Autodesk Inventor part; units mm, degrees
ref_plane "YZ Plane" through (0, 0, 0) normal (1, 0, 0) x (0, 1, 0)
ref_plane "XZ Plane" through (0, 0, 0) normal (0, 1, 0) x (-1, 0, 0)
ref_plane "XY Plane" through (0, 0, 0) normal (0, 0, 1) x (1, 0, 0)
sketch "Sketch1" plane through (0, 0, 0) normal (0, 0, 1) x (1, 0, 0)
  line L0 (0, 0) -> (19, 0)
  line L1 (19, 0) -> (19, 9)
  line L2 (19, 9) -> (0, 9)
  line L3 (0, 9) -> (0, 0)
  point P0 (9.5, 9)
  dimension "d0" = 19
  dimension "d1" = 9
extrude "Extrusion1" add sketch "Sketch1" along normal blind 3
sketch "Sketch2" plane through (0, 0, 3) normal (0, 0, 1) x (1, 0, 0)
  line L0 (19, 9) -> (0, 9)
  circle A0 centre (9.5, 7.5) radius 1.5
  line L1 (11, 6) -> (8, 6)
  line L2 (8, 6) -> (8, 9)
  line L3 (8, 9) -> (11, 9)
  line L4 (11, 9) -> (11, 6)
  line L5 (11, 6) -> (8, 9) construction
  line L6 (8, 6) -> (11, 9) construction
  line L7 (12, 7.5) -> (7, 7.5)
  line L8 (7, 7.5) -> (7, 9)
  line L9 (7, 9) -> (12, 9)
  line L10 (12, 9) -> (12, 7.5)
  line L11 (12, 7.5) -> (7, 9) construction
  line L12 (7, 7.5) -> (12, 9) construction
  line L13 (8, 7.5) -> (11, 7.5)
  line L14 (11, 7.5) -> (11, 6)
  line L15 (11, 6) -> (8, 6)
  line L16 (8, 6) -> (8, 7.5)
  point P0 (0, 0)
  point P1 (9.5, 8.25)
  dimension "d4" = 3
  dimension "d5" = 1.5
  dimension "d73" = 0.75
  dimension "d74" = 5
extrude "Extrusion2" add sketch "Sketch2" along normal blind 20 contours A0 L7 | A0 L7
sketch "Sketch10" plane through (0, 0, 0) normal (-1, 0, 0) x (0, 0, 1)
  line L0 (0, 0) -> (3, 0)
  line L1 (3, 9) -> (3, 0)
  line L2 (3, 0) -> (2, 0)
  line L3 (2, 0) -> (2, 6)
  line L4 (2, 6) -> (3, 6)
  line L5 (3, 6) -> (3, 0)
  line L6 (3, 0) -> (2, 1)
  line L7 (3, 0) -> (4.4142, 0) construction
  line L8 (2, 1) -> (3, 2)
  line L9 (3, 0) -> (3, 9)
  line L10 (3, 2) -> (2, 3)
  line L11 (2, 3) -> (3, 4)
  line L12 (2, 5) -> (3, 4)
  line L13 (2, 5) -> (3, 6)
  dimension "d23" = 1
  dimension "d24" = 6
  dimension "d25" = 135
  dimension "d26" = 90
extrude "Extrusion8" cut sketch "Sketch10" against normal up to next contours L6 L8 L1 | L10 L11 L1 | L12 L13 L1
sketch "Sketch11" plane through (0, 0, 0) normal (0, -1, 0) x (1, 0, 0)
  line L0 (0, 3) -> (9.5, 3)
  line L1 (0, 3) -> (19, 3)
  line L2 (19, 3) -> (19, 2)
  line L3 (19, 2) -> (8.5, 2)
  line L4 (0, 2) -> (0, 3)
  line L5 (0, 3) -> (0, 2)
  line L6 (0, 3) -> (1.4142, 3) construction
  line L7 (19, 3) -> (0, 3)
  line L8 (9.5, 3) -> (8.5, 2)
  line L9 (9.5, 3) -> (10.9142, 3) construction
  line L10 (10.5, 2) -> (8.5, 2)
  line L11 (9.5, 3) -> (10.5, 2)
  line L12 (10.5, 2) -> (8.5, 2)
  line L13 (8.5, 2) -> (0, 2)
  line L14 (7.5, 3) -> (8.5, 2)
  line L15 (8.5, 2) -> (6.5, 2)
  line L16 (7.5, 3) -> (6.5, 2)
  line L17 (5.5, 3) -> (6.5, 2)
  line L18 (6.5, 2) -> (4.5, 2)
  line L19 (5.5, 3) -> (4.5, 2)
  line L20 (3.5, 3) -> (4.5, 2)
  line L21 (4.5, 2) -> (2.5, 2)
  line L22 (3.5, 3) -> (2.5, 2)
  line L23 (12.5, 2) -> (10.5, 2)
  line L24 (11.5, 3) -> (12.5, 2)
  line L25 (11.5, 3) -> (10.5, 2)
  line L26 (14.5, 2) -> (12.5, 2)
  line L27 (13.5, 3) -> (14.5, 2)
  line L28 (13.5, 3) -> (12.5, 2)
  line L29 (16.5, 2) -> (14.5, 2)
  line L30 (15.5, 3) -> (16.5, 2)
  line L31 (15.5, 3) -> (14.5, 2)
  point P0 (0, 0)
  dimension "d30" = 135
  dimension "d33" = 2
  dimension "d40" = 2
extrude "Extrusion9" cut sketch "Sketch11" against normal blind 6 contours L0 L22 L13 L4 | L0 L19 L20 | L0 L16 L17 | L0 L8 L14 | L1 L25 L11 | L1 L28 L24 | L1 L31 L27 | L1 L2 L3 L30
fillet "Fillet2" radius 1 4 edges at (19, 0, 1) (19, 9, 1.5) (0, 0, 1) (0, 9, 1.5)
sketch "Sketch13" plane through (9.5, 7.5, 23) normal (0, 0, 1) x (1, 0, 0)
  line L0 (9.5, -6.5) -> (9.5, 0.5)
  arc A0 (8.5, -7.5) -> (9.5, -6.5) centre (8.5, -6.5) ccw
  line L1 (-8.5, -7.5) -> (8.5, -7.5)
  arc A1 (-9.5, -6.5) -> (-8.5, -7.5) centre (-8.5, -6.5) ccw
  line L2 (-9.5, 0.5) -> (-9.5, -6.5)
  arc A2 (-8.5, 1.5) -> (-9.5, 0.5) centre (-8.5, 0.5) ccw
  line L3 (8.5, 1.5) -> (-8.5, 1.5)
  arc A3 (9.5, 0.5) -> (8.5, 1.5) centre (8.5, 0.5) ccw
  point P0 (-9.5, -7.5)
extrude "Extrusion12" add sketch "Sketch13" along normal blind 4
sketch "Sketch14" plane through (9.5, 7.5, 27) normal (0, 0, 1) x (1, 0, 0)
  line L0 (-8.5, -7.5) -> (8.5, -7.5)
  circle A0 centre (0, -4.5) radius 1.65
  point P0 (-9.5, -7.5)
  dimension "d67" = 3
  dimension "d68" = 3.3
extrude "Extrusion13" cut sketch "Sketch14" against normal up to next
extrude "Extrusion14" add sketch "Sketch2" along normal up to next contours L4 A0 L0 | A0 L2 L0 | L4 L1 A0 | A0 L1 L2
extrude "Extrusion15" add sketch "Sketch2" along normal up to next contours L10 L7 L4 L0 | L4 A0 L0 | A0 L2 L0 | A0 L7 | L2 L7 L8 L0 picked at (9.5, 8)
extrude "Extrusion16" cut sketch "Sketch2" along normal up to surface (20 mm away) contours L4 L1 A0 | A0 L7 | A0 L1 L2 picked at (9.1091, 7.1883)
properties part number "clamp-base9x19mm-SampleH20-screwM4(Miracca)"
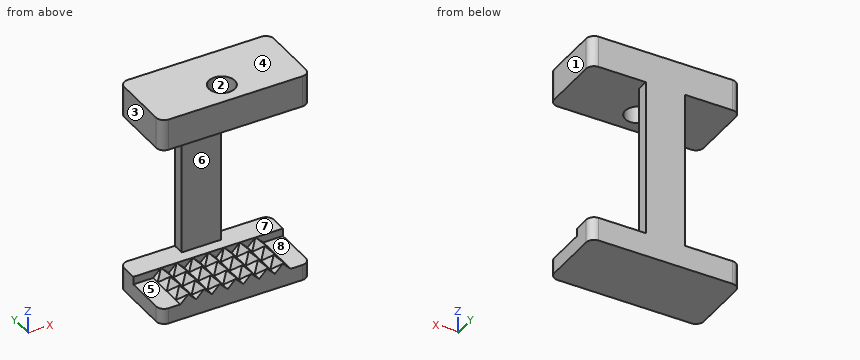
Here's how the part is built. I have some questions about the finished solid (model axes, mm). Face numbers are marked on the shaded views. A direction names the side the tool comes from. Coordinates: 2 decimals unless noted, no trailing zeros. Write each loop counter-clockwise with the first axis right and the second up, starting at its lowest first coordinate (ties: lowest second). Pieces come first, ordered by that corner, then holes. Notation, with made-up numbers: (13, 56.5) - (59, 56.5) arc R13 ccw to (59, 81.5) - close; hole circle Ø6 at (27, -11.5). An arc over 180 degrees is marked (long way). One line per item, written item: value.
1) We'd pull the mould along X, two halves only. Please class the marked faces 1, 2, 3 and 4: pulls with the +X half, pulls with the -X half, needs draft (parallel to the pull), parting line crosses it, or undercut.
Model answer:
face 1: pulls with the +X half
face 2: undercut
face 3: pulls with the -X half
face 4: needs draft
2) Suppose I cut it at A-A on z = 23.5. Write out the boundary of the cut face in (x, y), and give its area (3 significant figures).
Model answer:
outline: (0, 1) arc R1 ccw to (1, 0) - (18, 0) arc R1 ccw to (19, 1) - (19, 8) arc R1 ccw to (18, 9) - (1, 9) arc R1 ccw to (0, 8) - close; hole circle Ø3.3 at (9.5, 3)
area: 162 mm²
3) Suppose I cut it at B-B on z = 6.75. Write out the boundary of the cut face in (x, y), and give its area (3 significant figures).
Model answer:
outline: (7, 7.5) - (12, 7.5) - (12, 9) - (7, 9) - close
area: 7.50 mm²
4) I need wall thicknesses on line 1 along Z through (x, y) = (2.5, 7.5); line 2 along Z through (x, y) = (6.5, 3); line 3 along Y through (x, z) = (9.5, 25.7). Which ranges of each line are inside material? Lowest first, please.
Model answer:
line 1: z = 0 to 3, 23 to 27
line 2: z = 0 to 2, 23 to 27
line 3: y = 0 to 1.35, 4.65 to 9
5) On a 3-axis mill with a long thin cutter (end or side, diameter ignored), from which of +Z, -Z, +X, -X, +Y, -Y can I reach the whole of each face in a straight line? I mean the marked faces 5, 6, 7 and 8. Say none if no direction works.
Model answer:
face 5: -X, -Y
face 6: +X, -X, -Y
face 7: -Y
face 8: +X, -Y
6) I'm going to push flat-ended pins straight in: P1, Ø0.5, axis at x = 18, z = 2.5, coming from the -Y side; P2, Ø1.6, axis at y = 8, z = 14.5, coming from the -X side; P3, Ø2.5, axis at x = 9.5, z = 17, coming from the -Y side. Where does each tip first touch, or does it pass through?
Model answer:
P1: stops at y = 6
P2: stops at x = 7
P3: stops at y = 7.5
